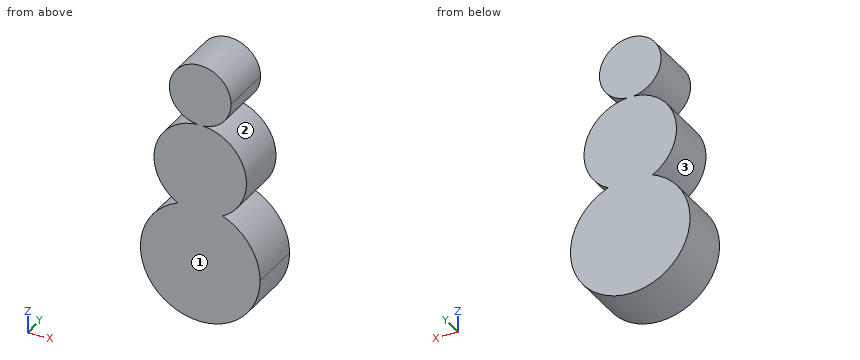
from build123d import *

# Parameters (mm, degrees)
F1_DEPTH = 25.4


with BuildPart() as f1:
    # F0 (on Front) → F1 (new body)
    with BuildSketch(Plane.XZ):
        with BuildLine():
            ThreePointArc((1.281621129, -14.6216553688), (10.8223525607, -9.9152429872), (14.6777163906, 0))
            ThreePointArc((14.6777163906, 0), (-9.9152429872, 10.8223525607), (-1.281621129, -14.6216553688))
            ThreePointArc((-1.281621129, -14.6216553688), (0, -14.5843201005), (1.281621129, -14.6216553688))
        make_face()
        with BuildLine():
            ThreePointArc((1.281621129, -14.6216553688), (0, -14.5843201005), (-1.281621129, -14.6216553688))
            ThreePointArc((-1.281621129, -14.6216553688), (0, -14.6777163906), (1.281621129, -14.6216553688))
        make_face()
        with BuildLine():
            ThreePointArc((1.281621129, -14.6216553688), (0, -14.6777163906), (-1.281621129, -14.6216553688))
            ThreePointArc((-1.281621129, -14.6216553688), (-21.4748376357, -31.7489642451), (-10.6053259906, -55.8936203584))
            ThreePointArc((-10.6053259906, -55.8936203584), (0, -53.8447494391), (10.6053259906, -55.8936203584))
            ThreePointArc((10.6053259906, -55.8936203584), (18.9498178248, -47.8078512952), (22.0160014308, -36.6003215313))
            ThreePointArc((22.0160014308, -36.6003215313), (16.0143762228, -21.4925727515), (1.281621129, -14.6216553688))
        make_face()
        with BuildLine():
            ThreePointArc((10.6053259906, -55.8936203584), (0, -53.8447494391), (-10.6053259906, -55.8936203584))
            ThreePointArc((-10.6053259906, -55.8936203584), (0, -58.6163229621), (10.6053259906, -55.8936203584))
        make_face()
        with BuildLine():
            ThreePointArc((10.6053259906, -55.8936203584), (0, -58.6163229621), (-10.6053259906, -55.8936203584))
            ThreePointArc((-10.6053259906, -55.8936203584), (-15.9483365423, -105.9028248142), (28.4719770071, -82.3167264462))
            ThreePointArc((28.4719770071, -82.3167264462), (23.586098368, -66.3683899038), (10.6053259906, -55.8936203584))
        make_face()
    extrude(amount=F1_DEPTH)


solid = f1.part
Input: part model. Units: mm. Frame: model coordinates. Face numbers are marked on the shaded views. Round coordinates to 2 decimals unless told otherwise and drop trailing zeros. Write each loop counter-clockwise with the first axis right and the second up, starting at its lowest first coordinate (ties: lowest second). Pieces come first, ordered by that corner, then holes.
1) Cut plane C-C (z = -62.5). Return the cut outline in (x, y).
2) Cut plane A-A (x = -6.5). Return the cut outline in (y, z).
3) Ray query, L1, parallel to Z at x = 13, y = -15.25; L2, parallel to Z at x = 5, y = -23; L3, parallel to Z at x = -8.5, y = -21.5. Return the intervals inside material, ascending.
4) Contact query for flat-ended pins moving along their axis: P1, Ø1.5, axis at y = -4.5, z = -86, coming from the -X side; P2, Ø8, axis at y = -23, z = -35, coming from the -X side; P3, Ø12, axis at x = -0.5, y = -19.5, coming from the +Z side; P4, Ø10, axis at x = -8, y = -15.5, coming from the +Z side. Output: stop coordinate, or through.
5) Cut plane D-D (x = 24). Return the cut outline in (y, z), then the cut area to 3 significant figures.
6) Draft query along Z for the marked faces 1, 2 and 3. Return one class per face: pulls with the +Z half, pulls with the -Z half, needs draft (parallel to the pull), parting line crosses it, or undercut.
7) Cut plane B-B (y = -23.75). Return the cut outline in (x, z).
Geometry says:
1. outline: (-20.44, -25.4) - (20.44, -25.4) - (20.44, 0) - (-20.44, 0) - close
2. outline: (-25.4, -110.04) - (0, -110.04) - (0, -15.57) - (-25.4, -15.57) - close; (-25.4, -13.16) - (0, -13.16) - (0, 13.16) - (-25.4, 13.16) - close
3. L1: z = -107.65 to -56.99, -54.37 to -18.83, -6.81 to 6.81
3. L2: z = -110.35 to -15.16, -13.8 to 13.8
3. L3: z = -109.49 to -16.29, -11.97 to 11.97
4. P1: stops at x = -28.32
4. P2: stops at x = -22.02
4. P3: stops at z = 14.68
4. P4: stops at z = 14.37
5. outline: (-25.4, -97.64) - (0, -97.64) - (0, -67) - (-25.4, -67) - close
5. area: 778 mm2
6. face 1: needs draft
6. face 2: undercut
6. face 3: undercut
7. outline: (-10.61, -55.89) arc R28.47 ccw (long way) to (10.61, -55.89) arc R22.02 ccw to (1.28, -14.62) arc R14.68 ccw (long way) to (-1.28, -14.62) arc R22.02 ccw to start
